Design review of the part shown in the three views and the two pictorial views. Dimensions are in mm from the part's minimum x, y and z. A direction names the side the tool comes from. Coordinates: 2 decimals unless noted, no trailing zeros. Loops run counter-clockwise (first coordinate to the right, second up) from the corner with the lowest first, then second, coordinate; pieces in that order, holes last. Notation, with made-up numbers: (76.5, -35) - (96.5, -35) arc R32 cw to (96.5, -1) - close; hole circle Ø11 at (33, 59). An arc over 180 degrees is marked (long way). One line per item, written item: value. Start each with the question number.
1. Take a section at A-A, the plane x = 7. State the section outline as (y, z) points.
2. For the marked faces 1 and 2, list the 3-axis set-ups (+Z, -Z, +X, -X, +Y, -Y) from which the entire face can be reached by the end or side of a thin tool; tool diameter is ignored.
3. To check wall thickness, follow line 1 (Z direction, x = 7, y = 1.25); line 2 (X direction, y = 5, z = 8). State the ranges of each line that lie inside material, in increasing order. Write a range as from..to.
4. Insertion check: pin 1 (2.5 mm diameter, centred on x = 7, z = 15, fed in from -Y); pin 2 (1 mm diameter, centred on x = 19.5, z = 17.5, fed in from +Y); pin 3 (3 mm diameter, centred on y = 24, z = 10.5, fed in from +X). Each pin has a flat end and moves straight along its axis. Give the tip position at first contact, or say it passes through.
5. Take a section at B-B, the plane y = 20. State the section outline as (x, z) points, and give its area (3 significant figures).
6. Take a section at D-D, the plane y = 7.5. State the section outline as (x, z) points, and give its area (3 significant figures).
7. Take a section at C-C, the plane z = 10. State the section outline as (x, y) points.
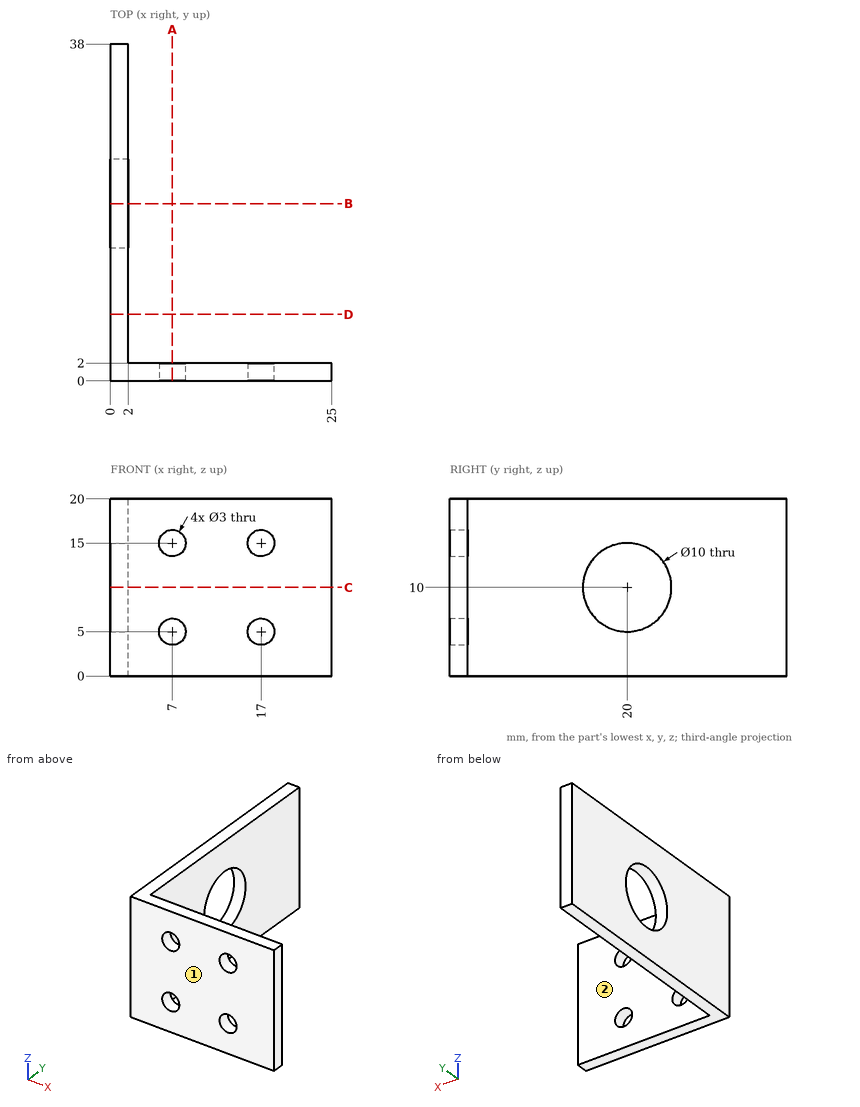
Solutions:
1. outline: (0, 0) - (2, 0) - (2, 3.5) - (0, 3.5) - close; (0, 6.5) - (2, 6.5) - (2, 13.5) - (0, 13.5) - close; (0, 16.5) - (2, 16.5) - (2, 20) - (0, 20) - close
2. face 1: +Z, -Z, +X, -X, -Y
2. face 2: +Z, -Z, +X, +Y
3. line 1: 0..3.5, 6.5..13.5, 16.5..20
3. line 2: 0..2
4. pin 1: through
4. pin 2: y = 2
4. pin 3: x = 2
5. outline: (0, 0) - (2, 0) - (2, 5) - (0, 5) - close; (0, 15) - (2, 15) - (2, 20) - (0, 20) - close
5. area: 20.0 mm2
6. outline: (0, 0) - (2, 0) - (2, 20) - (0, 20) - close
6. area: 40.0 mm2
7. outline: (0, 0) - (25, 0) - (25, 2) - (2, 2) - (2, 15) - (0, 15) - close; (0, 25) - (2, 25) - (2, 38) - (0, 38) - close
